from build123d import *

# Parameters (mm, degrees)
Y_KSEKLIK_EKSTR_ZYON1_DEPTH = 20
IZIM2_W                     = 100
IZIM2_H                     = 10
IZIM2_W_2                   = 10
IZIM2_H_2                   = 100
KES_EKSTR_ZYON1_DEPTH       = 12.5
IZIM4_R                     = 10
KES_EKSTR_ZYON2_DEPTH       = 230.5


with BuildPart() as part:
    # Çizim1 → Yükseklik-Ekstrüzyon1 (new body)
    with BuildSketch(Plane(origin=(0, 0, 0), x_dir=(1, 0, 0), z_dir=(0, 1, 0))):
        with BuildLine():
            Line((-41.125316458, 193.880424863), (168.874683542, 193.880424863))
            ThreePointArc((168.874683542, 193.880424863), (254.603263886, 68.880424863), (168.874683542, -56.119575137))
            Line((168.874683542, -56.119575137), (-41.125316458, -56.119575137))
            ThreePointArc((-41.125316458, -56.119575137), (-69.409587706, -44.403846384), (-81.125316458, -16.119575137))
            Line((-81.125316458, -16.119575137), (-81.125316458, 153.880424863))
            ThreePointArc((-81.125316458, 153.880424863), (-69.409587706, 182.16469611), (-41.125316458, 193.880424863))
        make_face()
    extrude(amount=Y_KSEKLIK_EKSTR_ZYON1_DEPTH)

    # Çizim2 → Kes-Ekstrüzyon1 (cut)
    with BuildSketch(Plane(origin=(0, 20, 0), x_dir=(1, 0, 0), z_dir=(0, 1, 0))):
        with Locations((53.874683542, 183.880424863)):
            Rectangle(IZIM2_W, IZIM2_H)
        with Locations((-71.125316458, 68.880424863)):
            Rectangle(IZIM2_W_2, IZIM2_H_2)
        with Locations((53.874683542, -46.119575137)):
            Rectangle(IZIM2_W, IZIM2_H)
    extrude(amount=-KES_EKSTR_ZYON1_DEPTH, mode=Mode.SUBTRACT)

    # Çizim4 → Kes-Ekstrüzyon2 (cut)
    with BuildSketch(Plane(origin=(0, 20, 0), x_dir=(1, 0, 0), z_dir=(0, 1, 0))):
        with Locations((68.874683542, 73.880424863)):
            Circle(IZIM4_R)
    extrude(amount=-KES_EKSTR_ZYON2_DEPTH, mode=Mode.SUBTRACT)


solid = part.part
The model under review builds one solid part; all positions refer to its coordinate system, in mm. A direction names the side the tool comes from. Coordinates: 2 decimals unless noted, no trailing zeros. Loops run counter-clockwise (first coordinate to the right, second up) from the corner with the lowest first, then second, coordinate; pieces in that order, holes last. Notation, with made-up numbers: (17.25, 84) -> (64.25, 84) arc R38 ccw to (64.25, 122) -> close; hole circle Ø10 at (69.5, 81.5). An arc over 180 degrees is marked (long way). Use a Markdown table: item, result. Add a question column.
1. To check wall thickness, follow line 1 (Z direction, x = 90, y = 9.75); line 2 (X direction, y = 15, z = -70.5); line 3 (X direction, y = 12.5, z = -65.5). State the ranges of each line that lie inside material, in increasing order.
2. Add section B-B on y = 15.25. Write out the cut boundary in (x, z).
3. Machinability: for faces 4 (the face through (65, 10, 56.12)), 5 (the face through (103.875, 14, 46)), which of the approach directions +Z, -Z, +X, -X, +Y, -Y give a long, thin tool a straight path to every point of the face, cutting with its end or side? Answer none if there is none.
4. Add section A-A on x = 38. Write out the cut boundary in (y, z), plus the area to 3 significant figures.
5. Add section C-C on z = -51. Write out the cut boundary in (x, y), plus the area to 3 significant figures.
6. Clearance check with flat-ended pins moving along their axes: pin 1 Ø5 at (x, z) = (77, -184) entering from +Y; pin 2 Ø2 at (x, z) = (192, -70.5) entering from -Y; pin 3 Ø11 at (y, z) = (11.5, -181.5) entering from -X; pin 4 Ø8 at (x, y) = (216, 15.5) entering from -Z. State where each tip first meets the part, or that it passes through.
7. Add section D-D on x = 221. Write out the cut boundary in (y, z), plus the area to 3 significant figures.
8. Draft analysis for pull direction Z (two halves, no side actions). For faces 1 (the face through (53, 7.5, -184)), 2 (the face through (89, 0, -71)), 3 (the face through (62, 10, -193.88)), state which applies: pulls with the +Z half, pulls with the -Z half, needs draft (parallel to the pull), parting line crosses it, or undercut.
Returned:
| question | item | result |
|---|---|---|
| 1 | line 1 | z = -193.88 to -188.88, -178.88 to 41.12, 51.12 to 56.12 |
| 1 | line 2 | x = -81.13 to -76.13, -66.13 to 59.46, 78.29 to 254.59 |
| 1 | line 3 | x = -81.13 to -76.13, -66.13 to 63.42, 74.33 to 254.56 |
| 2 | outline | (-81.13, -153.88) arc R40 ccw to (-41.13, -193.88) -> (168.87, -193.88) arc R133.99 ccw to (168.87, 56.12) -> (-41.13, 56.12) arc R40 ccw to (-81.13, 16.12) -> close; hole (-76.13, -118.88) -> (-66.13, -118.88) -> (-66.13, -18.88) -> (-76.13, -18.88) -> close; hole (3.87, -188.88) -> (103.87, -188.88) -> (103.87, -178.88) -> (3.87, -178.88) -> close; hole (3.87, 41.12) -> (103.87, 41.12) -> (103.87, 51.12) -> (3.87, 51.12) -> close; hole circle Ø20 at (68.87, -73.88) |
| 3 | face 4 | +Z, +X, -X, +Y, -Y |
| 3 | face 5 | +Y |
| 4 | outline | (0, -193.88) -> (20, -193.88) -> (20, -188.88) -> (7.5, -188.88) -> (7.5, -178.88) -> (20, -178.88) -> (20, 41.12) -> (7.5, 41.12) -> (7.5, 51.12) -> (20, 51.12) -> (20, 56.12) -> (0, 56.12) -> close |
| 4 | area | 4,750 mm² |
| 5 | outline | (-81.13, 0) -> (253.4, 0) -> (253.4, 20) -> (-66.13, 20) -> (-66.13, 7.5) -> (-76.13, 7.5) -> (-76.13, 20) -> (-81.13, 20) -> close |
| 5 | area | 6,570 mm² |
| 6 | pin 1 | stops at y = 7.5 |
| 6 | pin 2 | stops at y = 0 |
| 6 | pin 3 | stops at x = -74.45 |
| 6 | pin 4 | stops at z = -166.87 |
| 7 | outline | (0, -157.63) -> (20, -157.63) -> (20, 19.87) -> (0, 19.87) -> close |
| 7 | area | 3,550 mm² |
| 8 | face 1 | undercut |
| 8 | face 2 | needs draft |
| 8 | face 3 | pulls with the -Z half |
